```python
from build123d import *

# Parameters (mm, degrees)
BOSS_EXTRUDE2_DEPTH = 110
BOSS_EXTRUDE3_DEPTH = 5
SKETCH4_R           = 6
CUT_EXTRUDE1_DEPTH  = 5
SKETCH5_R           = 10
CUT_EXTRUDE2_DEPTH  = 5


with BuildPart() as part:
    # Sketch2 → Boss-Extrude2 (new body)
    with BuildSketch(Plane.XY):
        Polygon((0, 0), (0, 60), (10, 60), (10, 5), (120, 5), (120, 0), align=None)
    extrude(amount=BOSS_EXTRUDE2_DEPTH)

    # Sketch3 → Boss-Extrude3 (add)
    with BuildSketch(Plane.XZ):
        Polygon((60, 101.5), (0, 101.5), (0, 96.5), (120, 96.5), (120, 101.5), align=None)
        Polygon((120, 13.5), (0, 13.5), (0, 8.5), (60, 8.5), (120, 8.5), align=None)
    extrude(amount=BOSS_EXTRUDE3_DEPTH)

    # Sketch4 → Cut-Extrude1 (cut)
    with BuildSketch(Plane.ZY):
        with Locations((55, 30)):
            Circle(SKETCH4_R)
    extrude(amount=-CUT_EXTRUDE1_DEPTH, mode=Mode.SUBTRACT)

    # Sketch5 → Cut-Extrude2 (cut)
    with BuildSketch(Plane(origin=(10, 0, 0), x_dir=(0, 0, -1), z_dir=(1, 0, 0))):
        with Locations((-55, 30)):
            Circle(SKETCH5_R)
    extrude(amount=-CUT_EXTRUDE2_DEPTH, mode=Mode.SUBTRACT)


solid = part.part
```
Verification items for the finished model (mm, model axes). A direction names the side the tool comes from. Coordinates: 2 decimals unless noted, no trailing zeros. Loops run counter-clockwise (first coordinate to the right, second up) from the corner with the lowest first, then second, coordinate; pieces in that order, holes last. Notation, with made-up numbers: (-22.75, 63.5) -> (-6.75, 63.5) arc R16 cw to (-6.75, 93.5) -> close; hole circle Ø10 at (8.25, -11). An arc over 180 degrees is marked (long way). Answer in a Markdown table with one row per item. Add a question column.
1. Section check A-A, the plane z = 55. Enter the section's corners in (x, y).
2. Draft check along Z on faces 1 (the face through (59, -2, 8.5)), 2 (the face through (59, -5, 11)), 3 (the face through (59, -2, 96.5)). Enter one of: +Z half, -Z half, draft (parallel to the pull), parting line (faces both ways), or undercut.
3. Section check C-C, the plane x = 89. Enter the section's corners in (y, z).
4. Material ranges on probe 1 along Y at (x, z) = (8.7, 55); probe 2 along Y at (x, z) = (3.5, 55); probe 3 along X at (y, z) = (7.5, 82), recorded low to high. Write a range as [from, to].
5. Section check D-D, the plane z = 71. Enter the section's corners in (x, y).
6. Access from +Z, -Z, +X, -X, +Y, -Y to the whole of each face (thin tool, end or side, straight path). Record for faces 4 (the face through (61, 0, 4)), 5 (the face through (64, 5, 54)), 6 (the face through (61, 0, 54)), 7 (the face through (5, 23, 55)), 8 (the face through (61, -2, 101.5)).
7. Depth check by flat-ended pin: P1, Ø1.5, axis at y = 18.5, z = 76.5, coming from the +X side; P2, Ø3, axis at x = 77.5, z = 75.5, coming from the -Y side; P3, Ø6, axis at x = 105.5, y = 9.5, coming from the -Z side; P4, Ø10, axis at y = 39.5, z = 60.5, coming from the -X side. Enter the tip coordinate at first touch or a pass-through.
8. Section check B-B, the plane y = 30. Enter the section's corners in (x, z), then the cut area to 3 significant figures.
Derived:
| question | item | result |
|---|---|---|
| 1 | outline | (0, 0) -> (120, 0) -> (120, 5) -> (10, 5) -> (10, 20) -> (5, 20) -> (5, 24) -> (0, 24) -> close; (0, 36) -> (5, 36) -> (5, 40) -> (10, 40) -> (10, 60) -> (0, 60) -> close |
| 2 | face 1 | -Z half |
| 2 | face 2 | draft |
| 2 | face 3 | undercut |
| 3 | outline | (-5, 8.5) -> (0, 8.5) -> (0, 0) -> (5, 0) -> (5, 110) -> (0, 110) -> (0, 101.5) -> (-5, 101.5) -> (-5, 96.5) -> (0, 96.5) -> (0, 13.5) -> (-5, 13.5) -> close |
| 4 | probe 1 | y = [0, 20], [40, 60] |
| 4 | probe 2 | y = [0, 24], [36, 60] |
| 4 | probe 3 | x = [0, 10] |
| 5 | outline | (0, 0) -> (120, 0) -> (120, 5) -> (10, 5) -> (10, 60) -> (0, 60) -> close |
| 6 | face 4 | -Z, +X, -X, -Y |
| 6 | face 5 | +Z, -Z, +X, +Y |
| 6 | face 6 | +X, -X, -Y |
| 6 | face 7 | +X |
| 6 | face 8 | +Z, +X, -X, -Y |
| 7 | P1 | stops at x = 10 |
| 7 | P2 | stops at y = 0 |
| 7 | P3 | passes through |
| 7 | P4 | stops at x = 0 |
| 8 | outline | (0, 0) -> (10, 0) -> (10, 45) -> (5, 45) -> (5, 49) -> (0, 49) -> close; (0, 61) -> (5, 61) -> (5, 65) -> (10, 65) -> (10, 110) -> (0, 110) -> close |
| 8 | area | 940 mm² |
